Check sheet for the modelled part. Datum: model origin and axes. Units: mm. A direction names the side the tool comes from. Round coordinates to 2 decimals unless told otherwise and drop trailing zeros. Order: outer loops, then holes, each group sorted by start corner. A loop starts at its lowest first (then second) coordinate and runs counter-clockwise, first axis right, second up. Notation, with made-up numbers: (-28, -9) -> (-3, -9) arc R32 ccw to (-3, 29) -> close; hole circle Ø7 at (-13, -27.5). An arc over 180 degrees is marked (long way). Answer in a Markdown table with one row per item.
```python
from build123d import *

# Parameters (mm, degrees)
F1_DEPTH = 114.3
F2_R     = 9.525
F3_DEPTH = 114.301
F5_DEPTH = 5.6779
F6_R     = 12.7
F7_R     = 6.35
F8_DEPTH = 12.7


with BuildPart() as f1:
    # F0 (on Top) → F1 (new body)
    with BuildSketch(Plane.XY):
        Polygon((-31.75, 57.8231), (-57.15, 57.8231), (-57.15, -5.6769), (57.15, -5.6769), (57.15, 57.8231), (31.75, 57.8231), (31.75, 0), (-31.75, 0), align=None)
    extrude(amount=F1_DEPTH)

    # F2 (on face) → F3 (cut, through all)
    with BuildSketch(Plane(origin=(-57.15, 0, 0), x_dir=(0, -1, 0), z_dir=(-1, 0, 0))):
        with Locations((-26.0731, 25.4)):
            Circle(F2_R)
        with Locations((-26.0731, 88.9)):
            Circle(F2_R)
        with Locations((-26.0731, 57.15)):
            Circle(F2_R)
    extrude(amount=-F3_DEPTH, mode=Mode.SUBTRACT)

    # F4 (on face) → F5 (cut, through all)
    with BuildSketch(Plane(origin=(0, 0, 0), x_dir=(-1, 0, 0), z_dir=(0, 1, 0))):
        with BuildLine():
            Line((-31.75, 38.1), (-31.75, 0))
            Line((-31.75, 0), (31.75, 0))
            Line((31.75, 0), (31.75, 38.1))
            ThreePointArc((31.75, 38.1), (0, 69.85), (-31.75, 38.1))
        make_face()
    extrude(amount=-F5_DEPTH, mode=Mode.SUBTRACT)

    # F6
    f6_edges = [f1.edges().sort_by_distance(p)[0] for p in [
        (44.45, 57.8231, 114.3),
        (-44.45, 57.8231, 114.3),
    ]]
    fillet(f6_edges, radius=F6_R)

    # F7 (on face) → F8 (cut)
    with BuildSketch(Plane.XY.offset(114.3)):
        with Locations((-45.326655, 26.0731)):
            Circle(F7_R)
        with Locations((44.637317, 26.0731)):
            Circle(F7_R)
    extrude(amount=-F8_DEPTH, mode=Mode.SUBTRACT)


solid = f1.part
```
(1) Depth check by flat-ended pin: pin 1 Ø4 at (y, z) = (28.5, 62.5) entering from -X; pin 2 Ø4 at (x, y) = (-46, 24) entering from +Z; pin 3 Ø8 at (x, z) = (-6, 65.5) entering from +Y. Enter the tip coordinate at first touch or a pass-through.
Solutions:
| item | result |
|---|---|
| pin 1 | through |
| pin 2 | z = 101.6 |
| pin 3 | y = 0 |
(2) Section check C-C on y = 18. Give the number of separate pieces and of enclosed holes in the cut face, plus the area to 3 significant figures.
Solutions:
| item | result |
|---|---|
| separate pieces | 8 |
| enclosed holes | 0 |
| area | 4,270 mm^2 |
(3) Section check A-A on y = 2.5. Record the boundary of the cut face in (x, z).
Solutions:
| item | result |
|---|---|
| outline | (-57.15, 0) -> (-31.75, 0) -> (-31.75, 114.3) -> (-57.15, 114.3) -> close; (31.75, 0) -> (57.15, 0) -> (57.15, 114.3) -> (31.75, 114.3) -> close |
(4) Draft check along X on faces 1 (the flat face through (-44, 57.823, 50)), 2 (the flat face through (57.15, 26, 44)), 3 (the flat face through (45, 26, 101.6)). Enter one of: pulls with the +X half, pulls with the -X half, needs draft (parallel to the pull), parting line crosses it, or undercut.
Solutions:
| item | result |
|---|---|
| face 1 | needs draft |
| face 2 | pulls with the +X half |
| face 3 | undercut |
(5) Section check D-D on x = -47. Record the boundary of the cut face in (y, z) (3 decimals), plus the area to 3 significant figures.
Solutions:
| item | result |
|---|---|
| outline | (-5.677, 0) -> (57.823, 0) -> (57.823, 101.6) arc R12.7 ccw to (45.123, 114.3) -> (32.199, 114.3) -> (32.199, 101.6) -> (19.948, 101.6) -> (19.948, 114.3) -> (-5.677, 114.3) -> close; hole circle Ø19.05 at (26.073, 25.4); hole circle Ø19.05 at (26.073, 57.15); hole circle Ø19.05 at (26.073, 88.9) |
| area | 6,210 mm^2 |
(6) Scan lines: probe 1 along X at (y, z) = (34, 72.5); probe 2 along Y at (x, z) = (-50, 57); probe 3 along Z at (x, y) = (39, 26). Record each from-to range of solid material in increasing order. Write a range as from..to.
Solutions:
| item | result |
|---|---|
| probe 1 | -57.15..-31.75, 31.75..57.15 |
| probe 2 | -5.68..16.55, 35.6..57.82 |
| probe 3 | 0..15.88, 34.92..47.63, 66.67..79.38, 98.42..101.6 |
(7) Tool access check on faces 4 (the flat face through (-45, 26, 101.6)), 5 (the flat face through (-57.15, 27, 44)), 6 (the flat face through (0, 0, 93)). Record the directions out of +Z, -Z, +X, -X, +Y, -Y that give a thin tool (end or side, any length) a straight path to the whole face; none if there is none.
Solutions:
| item | result |
|---|---|
| face 4 | +Z |
| face 5 | +Z, -Z, -X, +Y, -Y |
| face 6 | +Z, -Z, +Y |
(8) Section check B-B on z = 25.4. Record the boundary of the cut face in (x, y).
Solutions:
| item | result |
|---|---|
| outline | (-57.15, -5.68) -> (-31.75, -5.68) -> (-31.75, 16.55) -> (-57.15, 16.55) -> close; (-57.15, 35.6) -> (-31.75, 35.6) -> (-31.75, 57.82) -> (-57.15, 57.82) -> close; (31.75, -5.68) -> (57.15, -5.68) -> (57.15, 16.55) -> (31.75, 16.55) -> close; (31.75, 35.6) -> (57.15, 35.6) -> (57.15, 57.82) -> (31.75, 57.82) -> close |
